```python
from build123d import *

# Parameters (mm, degrees)
F0_W     = 40
F0_H     = 5
F0_W_2   = 5
F0_R     = 1
F0_H_2   = 41
F1_DEPTH = 1
F2_DEPTH = 7
F3_DEPTH = 10


with BuildPart() as f1:
    # F0 (on Top) → F1 (new body)
    with BuildSketch(Plane.XY):
        with Locations((0, -23)):
            Rectangle(F0_W, F0_H)
        with Locations((0, 23)):
            Rectangle(F0_W, F0_H)
        with Locations((-22.5, 23)):
            Rectangle(F0_W_2, F0_H)
        with Locations((-22.5, 23)):
            Circle(F0_R, mode=Mode.SUBTRACT)
        with Locations((22.5, 23)):
            Rectangle(F0_W_2, F0_H)
        with Locations((22.5, 23)):
            Circle(F0_R, mode=Mode.SUBTRACT)
        with Locations((22.5, -23)):
            Rectangle(F0_W_2, F0_H)
        with Locations((22.5, -23)):
            Circle(F0_R, mode=Mode.SUBTRACT)
        with Locations((-22.5, -23)):
            Rectangle(F0_W_2, F0_H)
        with Locations((-22.5, -23)):
            Circle(F0_R, mode=Mode.SUBTRACT)
        with Locations((22.5, 0)):
            Rectangle(F0_W_2, F0_H_2)
        with Locations((-22.5, 23)):
            Circle(F0_R)
        with Locations((22.5, 23)):
            Circle(F0_R)
        with Locations((22.5, -23)):
            Circle(F0_R)
        with Locations((-22.5, -23)):
            Circle(F0_R)
    extrude(amount=F1_DEPTH)

    # F0 (on Top) → F2 (join)
    with BuildSketch(Plane.XY):
        with Locations((22.5, 23)):
            Rectangle(F0_W_2, F0_H)
        with Locations((22.5, 23)):
            Circle(F0_R, mode=Mode.SUBTRACT)
        with Locations((22.5, 23)):
            Circle(F0_R)
        with Locations((-22.5, 23)):
            Rectangle(F0_W_2, F0_H)
        with Locations((-22.5, 23)):
            Circle(F0_R, mode=Mode.SUBTRACT)
        with Locations((-22.5, 23)):
            Circle(F0_R)
        with Locations((22.5, -23)):
            Rectangle(F0_W_2, F0_H)
        with Locations((22.5, -23)):
            Circle(F0_R, mode=Mode.SUBTRACT)
        with Locations((22.5, -23)):
            Circle(F0_R)
        with Locations((-22.5, -23)):
            Rectangle(F0_W_2, F0_H)
        with Locations((-22.5, -23)):
            Circle(F0_R, mode=Mode.SUBTRACT)
        with Locations((-22.5, -23)):
            Circle(F0_R)
    extrude(amount=F2_DEPTH)

    # F0 (on Top) → F3 (join)
    with BuildSketch(Plane.XY):
        with Locations((22.5, 23)):
            Circle(F0_R)
        with Locations((-22.5, 23)):
            Circle(F0_R)
        with Locations((-22.5, -23)):
            Circle(F0_R)
        with Locations((22.5, -23)):
            Circle(F0_R)
    extrude(amount=F3_DEPTH)


solid = f1.part
```
CAD build for the part. Positions are in the model's coordinates, mm. A direction names the side the tool comes from. Coordinates: 2 decimals unless noted, no trailing zeros. Order: outer loops, then holes, each group sorted by start corner. A loop starts at its lowest first (then second) coordinate and runs counter-clockwise, first axis right, second up. Notation, with made-up numbers: (73.5, 79) - (90.5, 79) arc R10 ccw to (90.5, 85) - close; hole circle Ø11 at (-35, 57.25). An arc over 180 degrees is marked (long way). Use a Markdown table: item, result. Add a question column.
(1) Saw through at C-C (y = 23). Give the cut face in (x, z), then the cut area to 3 significant figures.
(2) Drill centre lines: line 1 along Y through (x, z) = (21, 4.75); line 2 along X through (y, z) = (22.5, 3.5). Where is each one in solid material? Low to high. Write a range as [from, to].
(3) Which spindle directions (+Z, -Z, +X, -X, +Y, -Y) get a long thin tool onto all of the face, cutting with end or side? Do faces 1 (the face through (22, 0, 1)), 2 (the face through (-21, -23, 7)), 3 (the face through (0, 23, 1)), 4 (the face through (-10.7, -20.5, 0.6)). Say none if no direction does.
(4) Saw through at A-A (x = 1.5). Give the cut face in (y, z), then the cut area to 3 significant figures.
(5) Pull direction X, two halves, no side cores. Call faces 5 (the face through (24, -23, 7)), 6 (the face through (-22.717, -23.976, 8.479)), 7 (the face through (-25, -23, 3)), 8 (the face through (22, 23, 10)): +X half, -X half, draft (parallel to the pull), parting line (faces both ways), or undercut.
(6) Saw through at D-D (z = 8). Give the cut face in (x, y).
(7) Saw through at B-B (x = 22.5). Give the cut face in (y, z), then the cut area to 3 significant figures.
(8) Flat gauge pins, fed straight in: pin 1 (2.5 mm diameter, centred on x = 8, y = -23.5, fed in from +Z); pin 2 (3.5 mm diameter, centred on x = 6, z = 4, fed in from -Y); pin 3 (0.8 mm diameter, centred on y = 3.5, z = 0.5, fed in from -X). Where does each tip first touch, or does it go through?
Solved:
| question | item | result |
|---|---|---|
| 1 | outline | (-25, 0) - (25, 0) - (25, 7) - (23.5, 7) - (23.5, 10) - (21.5, 10) - (21.5, 7) - (20, 7) - (20, 1) - (-20, 1) - (-20, 7) - (-21.5, 7) - (-21.5, 10) - (-23.5, 10) - (-23.5, 7) - (-25, 7) - close |
| 1 | area | 122 mm² |
| 2 | line 1 | y = [-25.5, -20.5], [20.5, 25.5] |
| 2 | line 2 | x = [-25, -20], [20, 25] |
| 3 | face 1 | +Z, +X, -X |
| 3 | face 2 | +Z |
| 3 | face 3 | +Z, +Y, -Y |
| 3 | face 4 | +Z, -Z, -X |
| 4 | outline | (-25.5, 0) - (-20.5, 0) - (-20.5, 1) - (-25.5, 1) - close; (20.5, 0) - (25.5, 0) - (25.5, 1) - (20.5, 1) - close |
| 4 | area | 10.0 mm² |
| 5 | face 5 | undercut |
| 5 | face 6 | undercut |
| 5 | face 7 | -X half |
| 5 | face 8 | draft |
| 6 | outline | circle Ø2 at (-22.5, -23); circle Ø2 at (-22.5, 23); circle Ø2 at (22.5, -23); circle Ø2 at (22.5, 23) |
| 7 | outline | (-25.5, 0) - (25.5, 0) - (25.5, 7) - (24, 7) - (24, 10) - (22, 10) - (22, 7) - (20.5, 7) - (20.5, 1) - (-20.5, 1) - (-20.5, 7) - (-22, 7) - (-22, 10) - (-24, 10) - (-24, 7) - (-25.5, 7) - close |
| 7 | area | 123 mm² |
| 8 | pin 1 | stops at z = 1 |
| 8 | pin 2 | passes through |
| 8 | pin 3 | stops at x = 20 |
